Source: CAD feature listing. Evaluate the final solid. Frame: model axes, mm. A direction names the side the tool comes from. Round coordinates to 2 decimals unless told otherwise and drop trailing zeros. Order: outer loops, then holes, each group sorted by start corner. A loop starts at its lowest first (then second) coordinate and runs counter-clockwise, first axis right, second up. Notation, with made-up numbers: M 53,-9 L 85,-9 A19 ccw 85,25 Z; hole C 85,-17.5 d11. An arc over 180 degrees is marked long. Answer as CSV lines item,"result". Start each with the question number.
Item 1: Set-up query: faces 1 (the face through (1.819, 0.9, 0.5)), 2 (the face through (-0.5, 5.581, 0.5)), 3 (the face through (20, 1, 0)). Return all of +Z, -Z, +X, -X, +Y, -Y with unobstructed straight access to the full face (end or side cutting, diameter ignored); none if empty.
Item 2: Section query C-C on y = -0.5. Return the cut outline in (x, z).
Item 3: Section query D-D on x = 20.25. Return the cut outline in (y, z).
Item 4: Line query: line 1 (X direction, y = -2.5, z = 0.75); line 2 (Z direction, x = 1.25, y = -1.25); line 3 (Y direction, x = 11, z = -1.75). Output: solid intervals per line, ascending. Write a range as [from, to].
Item 5: First-contact query: P1, Ø4, axis at x = 19.32, y = 2.83, coming from the -Z side; P2, Ø4, axis at x = 8, z = -1.5, coming from the +Y side. Flat tips, straight axial feed; report the tip coordinate or a pass-through.
Item 6: Section query A-A on z = -3.5. Return the cut outline in (x, y).
Item 7: Section query B-B on y = 2. Return the cut outline in (x, z), plus the area to 3 significant figures.
Item 8: Pull-direction query (Y, two-part tool) for faces 4 (the face through (17.82, 2.9, 0.49)), 5 (the face through (-0.51, 1.37, 0.49)), 6 (the face through (17.319, 1, 0.5)), 7 (the face through (10, -4.669, -1)); classes: +Y half, -Y half, draft (parallel to the pull), parting line (faces both ways), or undercut.
from build123d import *

# Parameters (mm, degrees)
ESBO_O1_R                = 1.5
RESSALTO_EXTRUS_O1_DEPTH = 1
ESBO_O2_W                = 25
ESBO_O2_H                = 1
RESSALTO_EXTRUS_O2_DEPTH = 6
ESBO_O3_R                = 1.75
CORTE_EXTRUS_O1_DEPTH    = 5


with BuildPart() as part:
    # Esboço1 → Ressalto-extrusão1 (new body)
    with BuildSketch(Plane.XY):
        Polygon((-2.930659551, 5.581459362), (-2.930659551, -4.668540638), (22.069340449, -4.668540638), (22.069340449, 5.581459362), (17.319340449, 5.581459362), (17.319340449, -3.668540638), (1.819340449, -3.668540638), (1.819340449, 5.581459362), align=None)
        with Locations((-0.180659551, 2.831459362)):
            Circle(ESBO_O1_R, mode=Mode.SUBTRACT)
        with Locations((19.319340449, 2.831459362)):
            Circle(ESBO_O1_R, mode=Mode.SUBTRACT)
    extrude(amount=RESSALTO_EXTRUS_O1_DEPTH)

    # Esboço2 → Ressalto-extrusão2 (add)
    with BuildSketch(Plane(origin=(0, 0, 0), x_dir=(-1, 0, 0), z_dir=(0, 0, -1))):
        with Locations((-9.569340449, -4.168540638)):
            Rectangle(ESBO_O2_W, ESBO_O2_H)
    extrude(amount=RESSALTO_EXTRUS_O2_DEPTH)

    # Esboço3 → Corte-extrusão1 (cut)
    with BuildSketch(Plane(origin=(0, -3.668540638, 0), x_dir=(1, 0, 0), z_dir=(0, 1, 0))):
        with Locations((9.627945133, 3.5)):
            Circle(ESBO_O3_R)
    extrude(amount=-CORTE_EXTRUS_O1_DEPTH, mode=Mode.SUBTRACT)


solid = part.part
Results:
1,face 1,"+Z, -Z, +Y"
1,face 2,"+Z, -Z, +X, -X, +Y"
1,face 3,"-Z, +X, -X, +Y"
2,outline,"M -2.93,0 L 1.82,0 L 1.82,1 L -2.93,1 Z; M 17.32,0 L 22.07,0 L 22.07,1 L 17.32,1 Z"
3,outline,"M -4.67,-6 L -3.67,-6 L -3.67,0 L 1.66,0 L 1.66,1 L -4.67,1 Z; M 4.01,0 L 5.58,0 L 5.58,1 L 4.01,1 Z"
4,line 1,"[-2.93, 1.82], [17.32, 22.07]"
4,line 2,"[0, 1]"
4,line 3,"[-4.67, -3.67]"
5,P1,"z = 0"
5,P2,"y = -3.67"
6,outline,"M -2.93,-4.67 L 7.88,-4.67 L 7.88,-3.67 L -2.93,-3.67 Z; M 11.38,-4.67 L 22.07,-4.67 L 22.07,-3.67 L 11.38,-3.67 Z"
7,outline,"M -2.93,0 L -1.43,0 L -1.43,1 L -2.93,1 Z; M 1.07,0 L 1.82,0 L 1.82,1 L 1.07,1 Z; M 17.32,0 L 18.07,0 L 18.07,1 L 17.32,1 Z; M 20.57,0 L 22.07,0 L 22.07,1 L 20.57,1 Z"
7,area,"4.51 mm^2"
8,face 4,"undercut"
8,face 5,"undercut"
8,face 6,"draft"
8,face 7,"-Y half"
